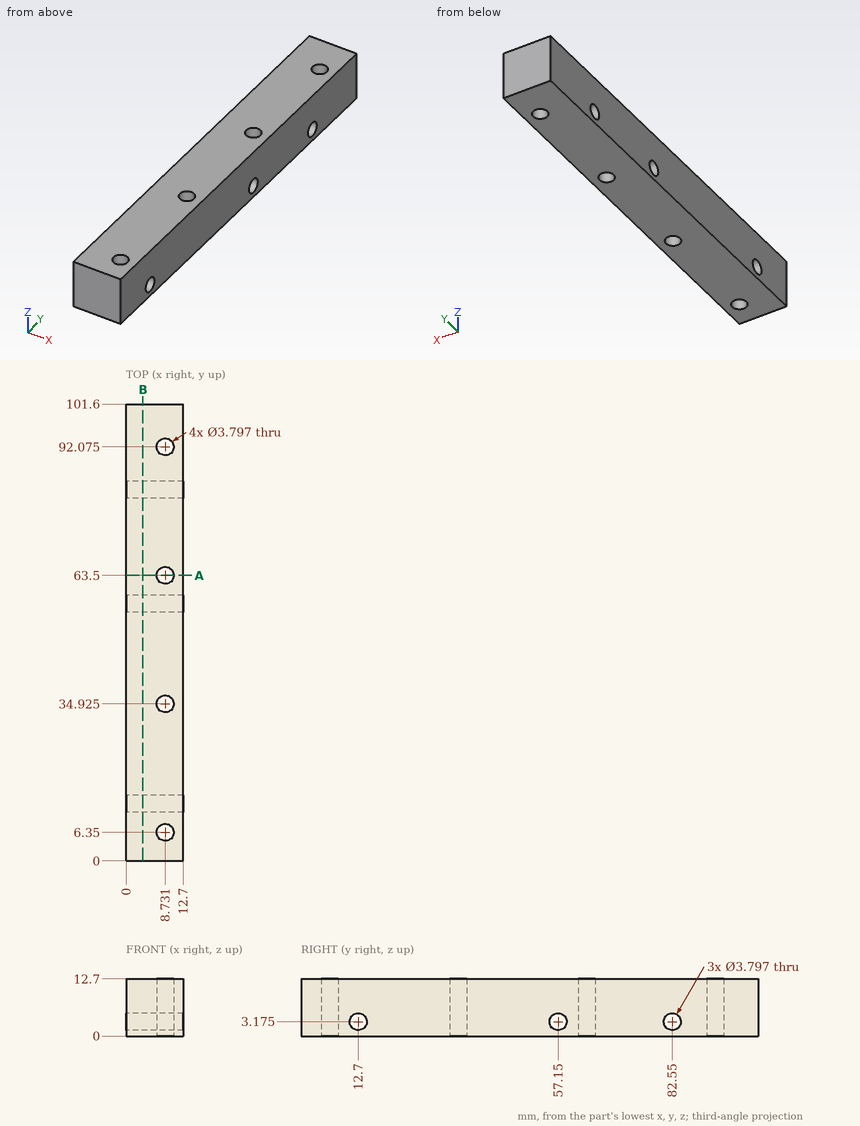
Job drawing, mm, ordinate dimensions from the low corner. One solid piece. Coordinates: 2 decimals unless noted, no trailing zeros. Order: outer loops, then holes, each group sorted by start corner. A loop starts at its lowest first (then second) coordinate and runs counter-clockwise, first axis right, second up. Notation, with made-up numbers: (43, 87.5) - (77, 87.5) arc R17 ccw to (77, 109.5) - close; hole circle Ø7 at (-16, 10.25). An arc over 180 degrees is marked (long way). Write each question's results on one line, items separated by ' | '. Start each with the question number.
Item 1: Band-saw the part on B-B on x = 3.75. State how many separate pieces and enclosed holes the cut face has, and give its area (3 significant figures).
Item 2: Flat gauge pin, fed straight in: pin 1 (6 mm diameter, centred on x = 8.73, y = 92.08, fed in from +Z). Where does the tip first touch, or does it go through?
Item 3: Wall check: probe 1 along Y at (x, z) = (8.75, 12.25); probe 2 along Y at (x, z) = (2, 3); probe 3 along Y at (x, z) = (10.25, 9.75) (1 decimal). Give the ranges that are in metal, low to high. Write a range as [from, to].
Item 4: Band-saw the part on A-A on y = 63.5. Write the cut outline in (x, z).
Numbers:
1) separate pieces: 1 | enclosed holes: 3 | area: 1,260 mm^2
2) pin 1: z = 12.7
3) probe 1: [0, 4.45], [8.25, 33.03], [36.82, 61.6], [65.4, 90.18], [93.97, 101.6] | probe 2: [0, 10.81], [14.59, 55.26], [59.04, 80.66], [84.44, 101.6] | probe 3: [0, 5.2], [7.5, 33.8], [36.1, 62.4], [64.6, 90.9], [93.2, 101.6]
4) outline: (0, 0) - (6.83, 0) - (6.83, 12.7) - (0, 12.7) - close; (10.63, 0) - (12.7, 0) - (12.7, 12.7) - (10.63, 12.7) - close
